```python
from build123d import *

# Parameters (mm, degrees)
F0_R     = 6.80000037
F1_DEPTH = 0.80000094
F2_R     = 6.0000007
F3_DEPTH = 3.999992
F4_R     = 2.999994
F5_DEPTH = 25.4
F6_R     = 5.6302817243
F6_R_2   = 3.4527411569
F7_DEPTH = 0.508
F8_R     = 2.999994
F8_R_2   = 2.3495
F9_DEPTH = 4.7999904


with BuildPart() as f1:
    # F0 (on Top) → F1 (new body)
    with BuildSketch(Plane.XY):
        with Locations((0, -1.4004084514)):
            Circle(F0_R)
    extrude(amount=F1_DEPTH)

    # F2 (on face) → F3 (join)
    with BuildSketch(Plane.XY.offset(0.80000094)):
        with Locations((0, -1.4004084514)):
            Circle(F2_R)
    extrude(amount=F3_DEPTH)

    # F4 (on face) → F5 (cut)
    with BuildSketch(Plane.XY.offset(4.79999294)):
        with Locations((0, -1.4004084514)):
            Circle(F4_R)
    extrude(amount=-F5_DEPTH, mode=Mode.SUBTRACT)

    # F6 (on face) → F7 (cut)
    with BuildSketch(Plane.XY.offset(4.79999294)):
        with Locations((0, -1.4004084514)):
            Circle(F6_R)
        with Locations((0, -1.4004084514)):
            Circle(F6_R_2, mode=Mode.SUBTRACT)
    extrude(amount=-F7_DEPTH, mode=Mode.SUBTRACT)

    # F8 (on face) → F9 (join)
    with BuildSketch(Plane(origin=(0, 0, 0), x_dir=(1, 0, 0), z_dir=(0, 0, -1))):
        with Locations((0, 1.4004084514)):
            Circle(F8_R)
        with Locations((0, 1.4004084514)):
            Circle(F8_R_2, mode=Mode.SUBTRACT)
    extrude(amount=-F9_DEPTH)


solid = f1.part
```
The model under review builds one solid part; all positions refer to its coordinate system, in mm. A direction names the side the tool comes from. Give positions to 0.01 mm unless a question says otherwise; leave off trailing zeros. Write each loop counter-clockwise with the first axis right and the second up, starting at its lowest first coordinate (ties: lowest second). Pieces come first, ordered by that corner, then holes. Notation, with made-up numbers: M -5.75,59.25 L 48.25,59.25 A4 cw 48.25,65.25 Z; hole C -34,9 d9. An arc over 180 degrees is marked long. Write item = value, one per line. Start each with the question number.
Q1. Mouldability with a two-part tool opening along Y and no side actions: class faces 1 (the face through (-1.301, -7.258, 2.772)), 2 (the face through (-3, -4, 4.292)), 3 (the face through (0, 2, 0)) as released by +Y, released by -Y, zero draft, split by the parting line, or undercut.
Q2. Clearance check with flat-ended pins moving along their axes: pin 1 (1.5 mm diameter, centred on x = 4.5, z = 1, fed in from -Y); pin 2 (3.5 mm diameter, centred on x = 0, y = -1.4, fed in from +Z); pin 3 (1.5 mm diameter, centred on x = -2.5, z = 2, fed in from +Y); pin 4 (1 mm diameter, centred on y = -4, z = 3.5, fed in from -X). State where each tip first meets the part, or that it passes through.
Q3. For line 1 (Y direction, x = 0, z = 4.4); line 2 (Y direction, x = 0, z = 2.75); line 3 (X direction, y = -1.5, z = 1.7), list the stretches that pass through material, from the lowest coordinate up.
Q4. We need section C-C (z = 4.55). State the section outline as (x, y) points.
Q5. We need section D-D (y = -6). State the section outline as (x, z) points.
Q6. Machinability: for faces 4 (the face through (-1.47, -8.04, 0.39)), 5 (the face through (-0.75, -4.77, 4.55)), which of the approach directions +Z, -Z, +X, -X, +Y, -Y give a long, thin tool a straight path to every point of the face, cutting with its end or side? Answer none if there is none.
Result set:
q1.face_1 = split by the parting line
q1.face_2 = undercut
q1.face_3 = zero draft
q2.pin_1 = -7.05
q2.pin_2 = through
q2.pin_3 = 4.34
q2.pin_4 = -5.62
q3.line_1 = -7.4 to -7.03, -4.85 to -3.75, 0.95 to 2.05, 4.23 to 4.6
q3.line_2 = -7.4 to -3.75, 0.95 to 4.6
q3.line_3 = -6 to -2.35, 2.35 to 6
q4.outline = C 0,-1.4 d12; C 0,-1.4 d6.91; hole C 0,-1.4 d11.26; hole C 0,-1.4 d4.7
q5.outline = M -5.01,0 L 5.01,0 L 5.01,0.8 L 3.85,0.8 L 3.85,4.8 L 3.25,4.8 L 3.25,4.29 L -3.25,4.29 L -3.25,4.8 L -3.85,4.8 L -3.85,0.8 L -5.01,0.8 Z
q6.face_4 = +Z, -Z
q6.face_5 = +Z
